from build123d import *

# Parameters (mm, degrees)
BOSS_EXTRUDE1_DEPTH = 28
BOSS_EXTRUDE2_DEPTH = 18
SKETCH4_R           = 3
BOSS_EXTRUDE3_DEPTH = 6


with BuildPart() as part:
    # Sketch1 → Boss-Extrude1 (new body)
    with BuildSketch(Plane.XY):
        Polygon((-78, 0), (0, 0), (0, 45.5), (-12.183101538, 49.547634765), (-27.397358961, 16.920554432), (-31.928897896, 19.033645741), (-16.714640473, 51.660726074), (-30.309257279, 58), (-41.500641075, 34), (-53.624640187, 8), (-78, 8), align=None)
    extrude(amount=BOSS_EXTRUDE1_DEPTH)

    # Sketch1<4> → Boss-Extrude2 (add)
    with BuildSketch(Plane.XY):
        Polygon((-78, 16), (-78, 8), (-53.624640187, 8), (-41.500641075, 34), (-54, 34), (-54, 16), align=None)
    extrude(amount=BOSS_EXTRUDE2_DEPTH)

    # Sketch4 → Boss-Extrude3 (add)
    with BuildSketch(Plane(origin=(16.80186773, 36.031721624, 0), x_dir=(0.9063077870366462, -0.4226182617407076, 0), z_dir=(0.4226182617407076, 0.9063077870366462, 0))):
        with Locations((-44.481375072, -21)):
            Circle(SKETCH4_R)
        with Locations((-44.481375072, -7)):
            Circle(SKETCH4_R)
    extrude(amount=BOSS_EXTRUDE3_DEPTH)


solid = part.part
The listing builds one solid part. Answer for the finished solid, in the listing's coordinates (mm). A direction names the side the tool comes from. Give positions to 0.01 mm unless a question says otherwise; leave off trailing zeros. Order: outer loops, then holes, each group sorted by start corner. A loop starts at its lowest first (then second) coordinate and runs counter-clockwise, first axis right, second up. Notation, with made-up numbers: (-20.75, -15) - (0.25, -15) arc R16 ccw to (0.25, 14) - close; hole circle Ø3 at (43, -31.5). An arc over 180 degrees is marked (long way). One line per item, written item: value. Start each with the question number.
1) Find the intervals of material crossed by L1, parallel to Y at x = -52, z = 15.5; L2, parallel to Z at x = -60, y = 10; L3, parallel to X at y = 30.5, z = 14, in increasing order.
2) A cutting plane is placed at D-D on z = 6. Give the vertices of the cut face in (x, y), then the cut area to 3 significant figures.
3) The mould has two halves that part along Z. Classify faces 1 (the face through (-20.8, 56.83, 4.47)), 2 (the face through (-66, 8, 23)), 3 (the face through (-60, 15, 18)), 4 (the face through (-31, 23, 0)): released by +Z, released by -Z, zero draft, split by the parting line, or undercut.
4) A cutting plane is placed at C-C on y = 32. Give the vertices of the cut face in (x, z).
5) A cutting plane is placed at A-A on z = 26. Give the vertices of the cut face in (x, y).
6) A cutting plane is placed at B-B on x = -73. Give the vertices of the cut face in (y, z).
7) A tool of negligible diameter and unlimited length cuts with its end or side. For faces 5 (the face through (-19.684, 33.462, 13.804)), 6 (the face through (-31, 23, 28)), 7 (the face through (-48, 34, 9)), from which of +Z, -Z, +X, -X, +Y, -Y can it reach the whole face along a straight path? Write none if from no direction.
8) Given pin 1 Ø1.5 at (x, z) = (-39.5, 9) entering from +Y; pin 2 Ø5 at (x, z) = (-14.5, 20) entering from +Y; pin 3 Ø8 at (x, y) = (-53, 26.5) entering from +Z, each flat-ended and moving along its own axis, determine where each tip first touches the part or whether it passes through.
Answer sheet:
1. L1: y = 0 to 34
1. L2: z = 0 to 18
1. L3: x = -54 to -26.58, -21.07 to 0
2. outline: (-78, 0) - (0, 0) - (0, 45.5) - (-12.18, 49.55) - (-27.4, 16.92) - (-31.93, 19.03) - (-16.71, 51.66) - (-20.95, 53.64) - (-18.41, 59.07) - (-23.54, 61.46) - (-26.08, 56.03) - (-30.31, 58) - (-41.5, 34) - (-54, 34) - (-54, 16) - (-78, 16) - close
2. area: 2,730 mm2
3. face 1: undercut
3. face 2: zero draft
3. face 3: released by +Z
3. face 4: released by -Z
4. outline: (-54, 0) - (-25.88, 0) - (-25.88, 28) - (-42.43, 28) - (-42.43, 18) - (-54, 18) - close; (-20.37, 0) - (0, 0) - (0, 28) - (-20.37, 28) - close
5. outline: (-78, 0) - (0, 0) - (0, 45.5) - (-12.18, 49.55) - (-27.4, 16.92) - (-31.93, 19.03) - (-16.71, 51.66) - (-30.31, 58) - (-53.62, 8) - (-78, 8) - close
6. outline: (0, 0) - (16, 0) - (16, 18) - (8, 18) - (8, 28) - (0, 28) - close
7. face 5: +Z, -Z
7. face 6: +Z, +X, -X, +Y, -Y
7. face 7: +Z, -Z, -X, +Y
8. pin 1: stops at y = 39.9
8. pin 2: stops at y = 51.79
8. pin 3: stops at z = 18
